```python
from build123d import *

# Parameters (mm, degrees)
F0_W      = 123.952538
F0_H      = 51.712212
F1_DEPTH  = 101.6
F2_R      = 33.878602
F2_R_2    = 21.701587
F3_DEPTH  = 38.1
F3_FACE_R = 21.701587
F4_DEPTH  = 2540


with BuildPart() as f1:
    # F0 (on Top) → F1 (new body)
    with BuildSketch(Plane.XY):
        Rectangle(F0_W, F0_H)
    extrude(amount=F1_DEPTH)

    # F2 (on face) → F3 (join)
    with BuildSketch(Plane.XZ.offset(25.856106)):
        with Locations((0, 50.8)):
            Circle(F2_R)
        with Locations((0, 50.8)):
            Circle(F2_R_2, mode=Mode.SUBTRACT)
    extrude(amount=F3_DEPTH)

    # F3_face (on face) → F4 (cut)
    with BuildSketch(Plane(origin=(0, -25.856106, 50.8), x_dir=(1, 0, 0), z_dir=(0, -1, 0))):
        Circle(F3_FACE_R)
    extrude(amount=-F4_DEPTH, mode=Mode.SUBTRACT)


solid = f1.part
```
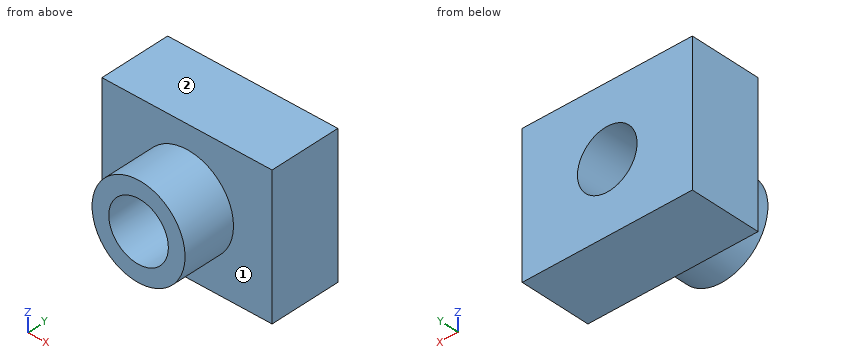
Geometry: final body of the model. Coordinates: model frame, mm. Face numbers are marked on the shaded views. A direction names the side the tool comes from. Coordinates: 2 decimals unless noted, no trailing zeros. Order: outer loops, then holes, each group sorted by start corner. A loop starts at its lowest first (then second) coordinate and runs counter-clockwise, first axis right, second up. Notation, with made-up numbers: (55, -35.75) -> (113, -35.75) arc R27 ccw to (113, 0.25) -> close; hole circle Ø4 at (83, 19). An arc over 180 degrees is marked (long way). Answer in a Markdown table with one row per item.
Item 1: Access query for the marked faces 1 and 2. Directions: +Z, -Z, +X, -X, +Y, -Y. A direction counts if a zero-diameter tool reaches every point of the face in a straight line with its end or side. Return the directions, or none.
Return value:
| item | result |
|---|---|
| face 1 | -Y |
| face 2 | +Z, +X, -X, +Y, -Y |
Item 2: Ray query, L1, parallel to Z at x = 0, y = -49.5; L2, parallel to Z at x = 0, y = -14; L3, parallel to Y at x = 37, z = 50. Return the intervals inside material, ascending.
Return value:
| item | result |
|---|---|
| L1 | z = 16.92 to 29.1, 72.5 to 84.68 |
| L2 | z = 0 to 29.1, 72.5 to 101.6 |
| L3 | y = -25.86 to 25.86 |
Item 3: Section C-C on y = 17.5. Output: boundary loops of the cut face in (x, z), plus the area to 3 significant figures.
Return value:
| item | result |
|---|---|
| outline | (-61.98, 0) -> (61.98, 0) -> (61.98, 101.6) -> (-61.98, 101.6) -> close; hole circle Ø43.4 at (0, 50.8) |
| area | 11,100 mm² |
Item 4: Contact query for flat-ended pins moving along their axis: P1, Ø1, axis at x = 35.5, y = -29, coming from the -Z side; P2, Ø2, axis at y = -49, z = 76, coming from the -X side; P3, Ø12, axis at y = -39, z = 63.5, coming from the +X side; P4, Ø5, axis at x = 32.5, y = -33.5, coming from the +Z side. Output: stop coordinate, or through.
Return value:
| item | result |
|---|---|
| P1 | passes through |
| P2 | stops at x = -23.71 |
| P3 | stops at x = 33.21 |
| P4 | stops at z = 66.54 |
Item 5: Section B-B on z = 50.8. Output: boundary loops of the cut face in (x, y), plus the area to 3 significant figures.
Return value:
| item | result |
|---|---|
| outline | (-61.98, -25.86) -> (-33.88, -25.86) -> (-33.88, -63.96) -> (-21.7, -63.96) -> (-21.7, 25.86) -> (-61.98, 25.86) -> close; (21.7, -63.96) -> (33.88, -63.96) -> (33.88, -25.86) -> (61.98, -25.86) -> (61.98, 25.86) -> (21.7, 25.86) -> close |
| area | 5,090 mm² |
Item 6: Section D-D on z = 11. Output: boundary loops of the cut face in (x, y), plus the area to 3 significant figures.
Return value:
| item | result |
|---|---|
| outline | (-61.98, -25.86) -> (61.98, -25.86) -> (61.98, 25.86) -> (-61.98, 25.86) -> close |
| area | 6,410 mm² |
Item 7: Section A-A on x = 0. Output: boundary loops of the cut face in (y, z).
Return value:
| item | result |
|---|---|
| outline | (-63.96, 16.92) -> (-25.86, 16.92) -> (-25.86, 0) -> (25.86, 0) -> (25.86, 29.1) -> (-63.96, 29.1) -> close; (-63.96, 72.5) -> (25.86, 72.5) -> (25.86, 101.6) -> (-25.86, 101.6) -> (-25.86, 84.68) -> (-63.96, 84.68) -> close |
